Input: part model. Units: mm. Frame: model coordinates. Face numbers are marked on the shaded views. A direction names the side the tool comes from. Coordinates: 2 decimals unless noted, no trailing zeros. Loops run counter-clockwise (first coordinate to the right, second up) from the corner with the lowest first, then second, coordinate; pieces in that order, holes last. Notation, with made-up numbers: M 40.5,22 L 51.5,22 A31 cw 51.5,52 Z; hole C -35.75,4 d11. An arc over 180 degrees is marked long. Use a Markdown table: item, result. Add a question column.
1. Section B-B on z = -15. Output: boundary loops of the cut face in (x, y), then the cut area to 3 significant figures.
2. Section C-C on x = -18. Output: boundary loops of the cut face in (y, z).
3. Set-up query: the marked faces 5, 6, 7, 8 and 9. Return all of +Z, -Z, +X, -X, +Y, -Y with unobstructed straight access to the full face (end or side cutting, diameter ignored); none if empty.
4. Section A-A on x = -30. Output: boundary loops of the cut face in (y, z).
5. Section D-D on z = -11.5. Output: boundary loops of the cut face in (x, y), then the cut area to 3 significant figures.
6. Draft query along X for the marked faces 1, 2, 3 and 4. Return one class per face: +X half, -X half, draft (parallel to the pull), parting line (faces both ways), or undercut.
7. Pin query (flat end, axial travel): pin 1 (4 mm diameter, centred on x = -19.5, y = 3.5, fed in from +Z); pin 2 (4 mm diameter, centred on x = -31, z = -15, fed in from +Y). Return the tip coordinate at first contact, or that it passes through.
8. Line query: L1, parallel to Z at x = -5, y = 5.75; L2, parallel to X at y = 3.25, z = -15; L3, parallel to X at y = 3.75, z = -15. Output: solid intervals per line, ascending. Write a range as [from, to].
```python
from build123d import *

# Parameters (mm, degrees)
SKETCH_2_W          = 36
SKETCH_2_H          = 30
EXTRUDE_1_DEPTH     = 10
SKETCH_3_R          = 6
CUT_EXTRUDE_1_DEPTH = 20
SKETCH_4_R          = 8.1
CUT_EXTRUDE_2_DEPTH = 5.2
SKETCH_5_R          = 1.45
CUT_EXTRUDE_3_DEPTH = 8
SKETCH_6_W          = 8
SKETCH_6_H          = 8
CUT_EXTRUDE_4_DEPTH = 8
CUT_EXTRUDE_5_DEPTH = 9.2
EXTRUDE_2_DEPTH     = 4


with BuildPart() as part:
    # 草图2 → 凸台-拉伸1 (new body)
    with BuildSketch(Plane(origin=(0, 0, 0), x_dir=(1, 0, 0), z_dir=(0, 1, 0))):
        with Locations((-18, 15)):
            Rectangle(SKETCH_2_W, SKETCH_2_H)
    extrude(amount=EXTRUDE_1_DEPTH)

    # 草图3 → 切除-拉伸1 (cut)
    with BuildSketch(Plane.XY):
        with Locations((-18, 0)):
            Circle(SKETCH_3_R)
    extrude(amount=-CUT_EXTRUDE_1_DEPTH, mode=Mode.SUBTRACT)

    # 草图4 → 切除-拉伸2 (cut)
    with BuildSketch(Plane.XY.offset(-20)):
        with Locations((-18, 0)):
            Circle(SKETCH_4_R)
    extrude(amount=-CUT_EXTRUDE_2_DEPTH, mode=Mode.SUBTRACT)

    # 草图5 → 切除-拉伸3 (cut)
    with BuildSketch(Plane.XZ):
        with Locations(Location((-31, -15, 0), (0, 0, 270))):
            Circle(SKETCH_5_R)
        with Locations(Location((-5, -15, 0), (0, 0, 90))):
            Circle(SKETCH_5_R)
    extrude(amount=-CUT_EXTRUDE_3_DEPTH, mode=Mode.SUBTRACT)

    # 草图6 → 切除-拉伸4 (cut)
    with BuildSketch(Plane.XZ.offset(-8)):
        with Locations((-32, -15)):
            Rectangle(SKETCH_6_W, SKETCH_6_H)
        with Locations((-4, -15)):
            Rectangle(SKETCH_6_W, SKETCH_6_H)
    extrude(amount=-CUT_EXTRUDE_4_DEPTH, mode=Mode.SUBTRACT)

    # 草图7 → 切除-拉伸5 (cut)
    with BuildSketch(Plane.XY):
        with BuildLine():
            Line((-26.1, 0), (-9.9, 0))
            ThreePointArc((-9.9, 0), (-18, 8.1), (-26.1, 0))
        make_face()
    extrude(amount=-CUT_EXTRUDE_5_DEPTH, mode=Mode.SUBTRACT)

    # 草图8 → 凸台-拉伸2 (add)
    with BuildSketch(Plane.XY):
        with BuildLine():
            Line((-12, 0), (-9.9, 0))
            ThreePointArc((-9.9, 0), (-18, 8.1), (-26.1, 0))
            Line((-26.1, 0), (-24, 0))
            ThreePointArc((-24, 0), (-18, 6), (-12, 0))
        make_face()
    extrude(amount=-EXTRUDE_2_DEPTH)


solid = part.part
```
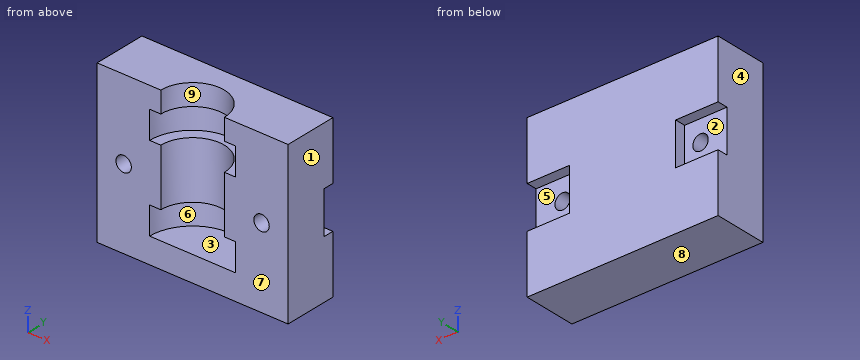
Answers below:
| question | item | result |
|---|---|---|
| 1 | outline | M -36,0 L -32.45,0 L -32.45,8 L -36,8 Z; M -29.55,0 L -24,0 A6 cw -12,0 L -6.45,0 L -6.45,8 L -8,8 L -8,10 L -28,10 L -28,8 L -29.55,8 Z; M -3.55,0 L 0,0 L 0,8 L -3.55,8 Z |
| 1 | area | 225 mm² |
| 2 | outline | M 0,-30 L 10,-30 L 10,0 L 6,0 L 6,-4 L 8.1,-4 L 8.1,-9.2 L 6,-9.2 L 6,-20 L 8.1,-20 L 8.1,-25.2 L 0,-25.2 Z |
| 3 | face 5 | +X, +Y |
| 3 | face 6 | -Y |
| 3 | face 7 | +Z, -Z, +X, -X, -Y |
| 3 | face 8 | -Z, +X, -X, +Y, -Y |
| 3 | face 9 | +Z, -Y |
| 4 | outline | M 0,-30 L 10,-30 L 10,-19 L 8,-19 L 8,-16.05 L 0,-16.05 Z; M 0,-13.95 L 8,-13.95 L 8,-11 L 10,-11 L 10,0 L 0,0 Z |
| 5 | outline | M -36,0 L -24,0 A6 cw -12,0 L 0,0 L 0,8 L -8,8 L -8,10 L -28,10 L -28,8 L -36,8 Z |
| 5 | area | 271 mm² |
| 6 | face 1 | +X half |
| 6 | face 2 | draft |
| 6 | face 3 | undercut |
| 6 | face 4 | -X half |
| 7 | pin 1 | stops at z = -25.2 |
| 7 | pin 2 | stops at y = 8 |
| 8 | L1 | z = [-30, -16.45], [-13.55, 0] |
| 8 | L2 | x = [-36, -32.45], [-29.55, -23.04], [-12.96, -6.45], [-3.55, 0] |
| 8 | L3 | x = [-36, -32.45], [-29.55, -22.68], [-13.32, -6.45], [-3.55, 0] |
